For this review, take the finished solid that the model builds, in its own axes (mm). Face numbers are marked on the shaded views. Round coordinates to 2 decimals unless told otherwise and drop trailing zeros. Write each loop counter-clockwise with the first axis right and the second up, starting at its lowest first coordinate (ties: lowest second). Pieces come first, ordered by that corner, then holes. Notation, with made-up numbers: M 64,46.25 L 81,46.25 A25 ccw 81,58.25 Z; hole C -37,12 d2. An arc over 180 degrees is marked long. Answer in a Markdown table with one row per item.
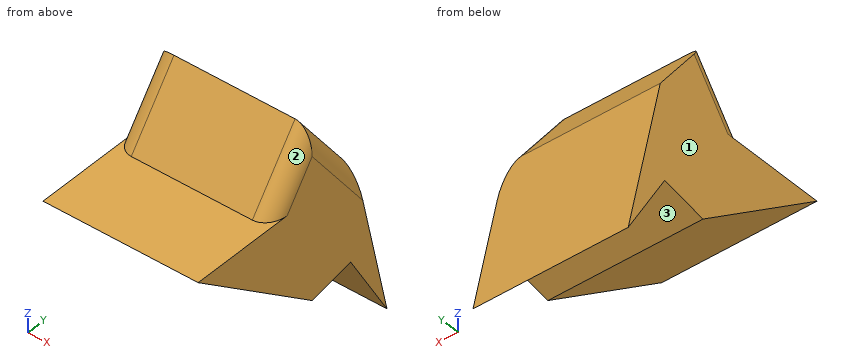
```python
from build123d import *

# Parameters (mm, degrees)
F1_DEPTH = 46.228
F2_R     = 5.08


with BuildPart() as f1:
    # F0 (on Right) → F1 (new body)
    with BuildSketch(Plane.YZ):
        Polygon((-14.183068, 10.637301), (0, 0), (13.716886, 2.820693), (26.699892, -19.010513), (15.24, 30.48), (0, 50.8), (-15.24, 30.48), (-40.64, 30.48), align=None)
    extrude(amount=F1_DEPTH)

    # F2
    f2_edges = [f1.edges().sort_by_distance(p)[0] for p in [
        (0, -7.62, 40.64),
        (46.228, -7.62, 40.64),
        (46.228, 7.62, 40.64),
    ]]
    fillet(f2_edges, radius=F2_R)


solid = f1.part
```
Q1. Mouldability with a two-part tool opening along Y and no side actions: class the marked faces 1, 2 and 3 as +Y half, -Y half, draft (parallel to the pull), parting line (faces both ways), or undercut.
Found:
| item | result |
|---|---|
| face 1 | draft |
| face 2 | -Y half |
| face 3 | undercut |
Q2. Take a section at A-A (x = 35). State the section outline as (y, z) points.
Found:
| item | result |
|---|---|
| outline | M -40.64,30.48 L 0,0 L 13.72,2.82 L 26.7,-19.01 L 15.24,30.48 L 0,50.8 L -15.24,30.48 Z |
Q3. Insertion check: P1, Ø8, axis at x = 11, y = -17, coming from the -Z side; P2, Ø1, axis at x = 37, z = 11, coming from the -Y side; P3, Ø2, axis at x = 8.5, y = 4, coming from the +Z side. Each pin has a flat end and moves straight along its axis. Give the tip position at first contact, or say it passes through.
Found:
| item | result |
|---|---|
| P1 | z = 9.75 |
| P2 | y = -15.33 |
| P3 | z = 46.8 |
Q4. Take a section at C-C (z = -9.5). State the section outline as (x, y) points.
Found:
| item | result |
|---|---|
| outline | M 0,21.04 L 46.23,21.04 L 46.23,24.5 L 0,24.5 Z |
Q5. Take a section at D-D (x = 3.5). State the section outline as (y, z) points, then the cut area to 3 significant figures.
Found:
| item | result |
|---|---|
| outline | M -40.64,30.48 L 0,0 L 13.72,2.82 L 26.7,-19.01 L 15.24,30.48 L 0.16,50.59 L -14.93,30.48 Z |
| area | 1,540 mm² |
Q6. Take a section at B-B (y = -21). State the section outline as (x, z) points, then the cut area to 3 significant figures.
Found:
| item | result |
|---|---|
| outline | M 0,15.75 L 46.23,15.75 L 46.23,30.48 L 0,30.48 Z |
| area | 681 mm² |
Q7. For probe 1 along Z at (x, y) = (25, 10); probe 2 along Z at (x, y) = (38, -31); probe 3 along Y at (x, z) = (12.5, 42.5) (3 decimals), list the stretches that pass through material, from the lowest coordinate up.
Found:
| item | result |
|---|---|
| probe 1 | 2.06 to 37.47 |
| probe 2 | 23.25 to 30.48 |
| probe 3 | -6.225 to 6.225 |
